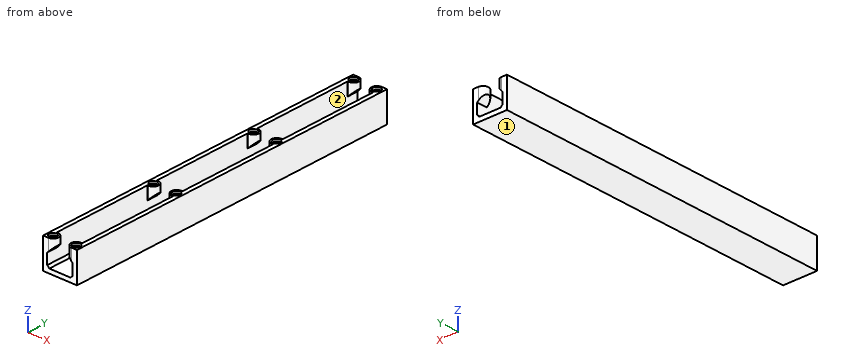
Autodesk Fusion 360 part; units mm, degrees
sketch "3D-printed conduit outline" plane through (0, 0, 0) normal (0, 1, 0) x (1, 0, 0)
  line L0 (0, 0) -> (16, 0)
  line L1 (16, 0) -> (16, -14)
  line L2 (16, -14) -> (0, -14)
  line L3 (0, -14) -> (0, 0)
  line L4 (2, -14) -> (14, -14)
  line L5 (14, -14) -> (14, -2)
  line L6 (14, -2) -> (2, -2)
  line L7 (2, -2) -> (2, -14)
  dimension "d8" = 14
  dimension "d9" = 16
  dimension "d10" = 2
  dimension "d11" = 2
  dimension "d12" = 2
extrude "Extrude1" add sketch "3D-printed conduit outline" along normal blind 161 contours L0 L1 L2 L3 L5 L6 L7
sketch "Magnet holders" plane through (0, 0, 14) normal (0, 0, 1) x (-1, 0, 0)
  line L0 (0, 0) -> (-2, 0)
  line L1 (-2, 0) -> (-2, -161)
  line L2 (-2, -161) -> (0, -161)
  line L3 (0, -161) -> (0, 0)
  line L4 (-14, 0) -> (-16, 0)
  line L5 (-16, 0) -> (-16, -161)
  line L6 (-16, -161) -> (-14, -161)
  line L7 (-14, -161) -> (-14, 0)
  circle A0 centre (-2.5, -2.5) radius 2.5
  circle A1 centre (-2.5, -2.5) radius 1.75
  line L8 (-14, 0) -> (-2, 0)
  line L9 (0, 0) -> (-2.5, 0)
  line L10 (-2.5, 0) -> (-2.5, -5)
  line L11 (-2.5, -5) -> (0, -5)
  line L12 (0, -5) -> (0, 0)
  circle A2 centre (-13.5, -2.5) radius 2.5
  circle A3 centre (-13.5, -2.5) radius 1.75
  line L13 (-16, 0) -> (-13.5, 0)
  line L14 (-13.5, 0) -> (-13.5, -5)
  line L15 (-13.5, -5) -> (-16, -5)
  line L16 (-16, -5) -> (-16, 0)
  circle A4 centre (-2.5, -54.5) radius 1.75
  circle A5 centre (-2.5, -54.5) radius 2.5
  line L17 (-2.5, -52) -> (-2.5, -57)
  line L18 (-2.5, -57) -> (0, -57)
  line L19 (0, -57) -> (0, -52)
  line L20 (0, -52) -> (-2.5, -52)
  circle A6 centre (-13.5, -54.5) radius 1.75
  circle A7 centre (-13.5, -54.5) radius 2.5
  line L21 (-13.5, -52) -> (-13.5, -57)
  line L22 (-13.5, -57) -> (-16, -57)
  line L23 (-16, -57) -> (-16, -52)
  line L24 (-16, -52) -> (-13.5, -52)
  circle A8 centre (-2.5, -106.5) radius 1.75
  circle A9 centre (-2.5, -106.5) radius 2.5
  line L25 (-2.5, -104) -> (-2.5, -109)
  line L26 (-2.5, -109) -> (0, -109)
  line L27 (0, -109) -> (0, -104)
  line L28 (0, -104) -> (-2.5, -104)
  circle A10 centre (-13.5, -106.5) radius 1.75
  circle A11 centre (-13.5, -106.5) radius 2.5
  line L29 (-13.5, -104) -> (-13.5, -109)
  line L30 (-13.5, -109) -> (-16, -109)
  line L31 (-16, -109) -> (-16, -104)
  line L32 (-16, -104) -> (-13.5, -104)
  circle A12 centre (-2.5, -158.5) radius 1.75
  circle A13 centre (-2.5, -158.5) radius 2.5
  line L33 (-2.5, -156) -> (-2.5, -161)
  line L34 (-2.5, -161) -> (0, -161)
  line L35 (0, -161) -> (0, -156)
  line L36 (0, -156) -> (-2.5, -156)
  circle A14 centre (-13.5, -158.5) radius 1.75
  circle A15 centre (-13.5, -158.5) radius 2.5
  line L37 (-13.5, -156) -> (-13.5, -161)
  line L38 (-13.5, -161) -> (-16, -161)
  line L39 (-16, -161) -> (-16, -156)
  line L40 (-16, -156) -> (-13.5, -156)
  dimension "d15" = 5
  dimension "d16" = 3.5
  dimension "d17" = 5
  dimension "d18" = 3.5
  dimension "d21" = 0
  dimension "d22" = -156
extrude "Extrude2" add sketch "Magnet holders" against normal blind 3 contours A2 A3 L14 | L7 A2 A3 L14 | L7 L8 A2 L13 | L1 A0 L8 L9 | L1 A0 A1 L10 | A0 A1 L10 | L1 A0 A1 L10 | L1 A0 L11 | L1 A1 L10 | A1 L10 | L7 A3 L14 | A3 L14 | L1 A5 L20 | L7 A2 L15 | L7 A2 A3 L14 | L1 A4 A5 L17 | L1 A4 A5 L17 | L1 A5 L18 | A4 A5 L17 | L1 A4 L17 | A4 L17 | L7 A7 L24 | L1 A9 L28 | L7 A6 A7 L21 | A6 A7 L21 | L1 A8 A9 L25 | L1 A8 A9 L25 | L1 A9 L26 | A8 A9 L25 | L7 A6 L21 | A6 L21 | L7 A7 L22 | L7 A6 A7 L21 | L1 A8 L25 | A8 L25 | L1 A13 L36 | L7 A11 L32 | L1 A12 A13 L33 | L1 A12 A13 L33 | L1 A13 L34 | A12 A13 L33 | L7 A10 A11 L29 | L7 A11 L30 | L7 A10 A11 L29 | A10 A11 L29 | L1 A12 L33 | A12 L33 | L7 A10 L29 | A10 L29 | L7 A15 L40 | L7 A14 A15 L37 | L7 A15 L38 | L7 A14 A15 L37 | A14 A15 L37 | L7 A14 L37 | A14 L37
extrude "Extrude3" cut sketch "Magnet holders" against normal blind 1 contours L1 A1 | L1 A1 L10 | A1 L10 | L7 A3 L14 | A3 L14 | L7 A3 | L1 A4 | L1 A4 L17 | A4 L17 | L7 A6 L21 | L7 A6 | A6 L21 | L1 A8 | L1 A8 L25 | A8 L25 | L1 A12 | L1 A12 L33 | A12 L33 | L7 A10 L29 | L7 A10 | A10 L29 | L7 A14 L37 | L7 A14 | A14 L37
chamfer "Chamfer1" distance 1 angle 45 2 edges at (2, 80.5, 2) (14, 80.5, 2)
chamfer "Chamfer2" distance 2.9999 angle 45 8 edges at (2, 2.5, 11) (2, 54.5, 11) (2, 106.5, 11) (2, 158.5, 11) (14, 2.5, 11) (14, 54.5, 11) (14, 106.5, 11) (14, 158.5, 11)
equation "conduit_length = 161 mm"
equation "conduit_width = 16 mm"
equation "conduit_height = 16 mm"
equation "conduit_wall_thickness = 2 mm"
equation "magnet_diameter = 3 mm"
equation "magnet_height = 1 mm"
equation "d8 = conduit_height - conduit_wall_thickness"
equation "d9 = conduit_width"
equation "d10 = conduit_wall_thickness"
equation "d11 = conduit_wall_thickness"
equation "d12 = conduit_wall_thickness"
equation "d13 = conduit_length"
equation "d15 = magnet_diameter + 2 mm"
equation "d16 = magnet_diameter + 0.5 mm"
equation "d17 = magnet_diameter + 2 mm"
equation "d18 = magnet_diameter + 0.5 mm"
equation "d22 = -conduit_length + ( magnet_diameter + 2 mm )"
equation "d23 = -( magnet_height + 2 mm )"
The listing builds one solid part. Answer for the finished solid, in the listing's coordinates (mm). Face numbers are marked on the shaded views. Round coordinates to 2 decimals unless told otherwise and drop trailing zeros. Loops run counter-clockwise (first coordinate to the right, second up) from the corner with the lowest first, then second, coordinate; pieces in that order, holes last. Notation, with made-up numbers: (71.5, 2.25) -> (123.5, 2.25) arc R10 ccw to (123.5, 11.25) -> close; hole circle Ø6 at (80.5, 21). An arc over 180 degrees is marked (long way). Use one line per item in the form item = value.
1. For a pull along Y with two mould halves and no side action, classify the marked faces 1 and 2 as released by +Y, released by -Y, zero draft, split by the parting line, or undercut.
Answer key:
face_1 = zero draft
face_2 = undercut
2. The part is cut by section A-A on y = 115.5. Determine the outline of the cut face in (x, z), and give its area (3 significant figures).
Answer key:
outline = (0, 0) -> (16, 0) -> (16, 14) -> (14, 14) -> (14, 3) -> (13, 2) -> (3, 2) -> (2, 3) -> (2, 14) -> (0, 14) -> close
area = 81.0 mm²
3. Find the intervals of material crossed by probe 1 along X at (y, z) = (2.5, 13.7); probe 2 along X at (y, z) = (123, 3.5); probe 3 along Z at (x, y) = (3.5, 88), in increasing order. Write a range as [from, to].
Answer key:
probe_1 = [0, 0.75], [4.25, 5], [11, 11.75], [15.25, 16]
probe_2 = [0, 2], [14, 16]
probe_3 = [0, 2]
4. Flat-ended cylindrical pins translate along their axes: pin 1 Ø1 at (x, y) = (7.5, 36.5) entering from +Z; pin 2 Ø1.8 at (x, y) = (2.5, 54.5) entering from +Z. Find the tip coordinate at first contact, or state that the pin passes through.
Answer key:
pin_1 = 2
pin_2 = 13
